Autodesk Inventor part; units mm, degrees
ref_plane "YZ Plane" through (0, 0, 0) normal (1, 0, 0) x (0, 1, 0)
ref_plane "XZ Plane" through (0, 0, 0) normal (0, 1, 0) x (-1, 0, 0)
ref_plane "XY Plane" through (0, 0, 0) normal (0, 0, 1) x (1, 0, 0)
sketch "Sketch1" plane through (0, 0, 0) normal (0, 1, 0) x (-1, 0, 0)
  line L0 (0, 0) -> (304.8, 0)
  line L1 (304.8, 0) -> (304.8, -190.5)
  line L2 (304.8, -190.5) -> (0, -190.5)
  line L3 (0, -190.5) -> (0, 0)
  dimension "d0" = 304.8
  dimension "d1" = 190.5
extrude "Extrusion1" add sketch "Sketch1" along normal blind 1.6
sketch "Sketch2" plane through (0, 1.6, 0) normal (0, 1, 0) x (1, 0, 0)
  line L0 (-304.8, 0) -> (0, 0)
  line L1 (-140.97, 0) -> (-140.97, 10.16)
  line L2 (-140.97, 0) -> (-130.81, 0) construction
  line L3 (-140.97, 10.16) -> (-140.97, 33.02)
  line L4 (-140.97, 33.02) -> (-255.8376, 33.02)
  line L5 (-140.97, 10.16) -> (-95.25, 10.16)
  line L6 (-95.25, 10.16) -> (-16.51, 10.16)
  line L7 (-16.51, 10.16) -> (-16.51, 165.1)
  line L8 (-140.97, 10.16) -> (-140.97, 165.1)
  line L9 (0, 0) -> (0, 190.5)
  line L10 (-16.51, 165.1) -> (-295.91, 165.1)
  line L11 (-295.91, 165.1) -> (-295.91, 33.02)
  line L12 (-295.91, 33.02) -> (-255.8376, 33.02)
  circle A0 centre (-295.91, 33.02) radius 2.54
  circle A1 centre (-295.91, 165.1) radius 2.54
  circle A2 centre (-140.97, 165.1) radius 2.54
  circle A3 centre (-16.51, 165.1) radius 2.54
  circle A4 centre (-16.51, 10.16) radius 2.54
  circle A5 centre (-140.97, 10.16) radius 2.54
  point P0 (-299.72, 0)
  point P1 (-5.08, 0)
  point P2 (0, 5.08)
  point P3 (0, 185.42)
  dimension "d5" = 10.16
  dimension "d6" = 90
  dimension "d8" = 78.74
  dimension "d9" = 45.72
  dimension "d10" = 22.86
  dimension "d11" = 154.94
  dimension "d12" = 154.94
  dimension "d13" = 16.51
  dimension "d14" = 279.4
  dimension "d15" = 5.08
  dimension "d16" = 5.08
  dimension "d17" = 5.08
  dimension "d18" = 5.08
  dimension "d19" = 5.08
  dimension "d20" = 5.08
extrude "Extrusion2" cut sketch "Sketch2" against normal through all contours A5 L3 L1 | L1 L5 A5 | L3 A5 L5 | A2 L10 L8 | L8 L10 A2 | A4 L7 L6 | L6 L7 A4 | A0 L11 L12 | L12 L11 A0 | L10 A2 | A1 L11 L10 | L10 L11 A1 | A3 L7 L10 | L10 L7 A3
sketch "Sketch3" plane through (0, 0, 0) normal (0, 1, 0) x (-1, 0, 0)
  circle A0 centre (16.51, -165.1) radius 2.54
  circle A1 centre (16.51, -165.1) radius 2.3813
  circle A2 centre (16.51, -10.16) radius 2.54
  circle A3 centre (16.51, -10.16) radius 2.3813
  circle A4 centre (140.97, -10.16) radius 2.54
  circle A5 centre (140.97, -10.16) radius 2.3813
  circle A6 centre (295.91, -33.02) radius 2.54
  circle A7 centre (295.91, -33.02) radius 2.3813
  circle A8 centre (295.91, -165.1) radius 2.54
  circle A9 centre (295.91, -165.1) radius 2.3813
  circle A10 centre (140.97, -165.1) radius 2.54
  circle A11 centre (140.97, -165.1) radius 2.3813
  point P0 (0, 0)
extrude "Extrusion3" add sketch "Sketch3" along normal blind 2.54 contours A0 | A1 | A2 | A3 | A4 | A5 | A6 | A7 | A8 | A9 | A10 | A11
sketch "Sketch4" plane through (-140.97, 2.54, -10.16) normal (0, 1, 0) x (1, 0, 0)
  circle A0 centre (0, 0) radius 1.9812
  circle A1 centre (-154.94, 22.86) radius 2.54
  circle A2 centre (-154.94, 22.86) radius 1.9812
  circle A3 centre (0, 154.94) radius 2.54
  circle A4 centre (0, 154.94) radius 1.9812
  circle A5 centre (124.46, 154.94) radius 2.54
  circle A6 centre (124.46, 154.94) radius 1.9812
  circle A7 centre (-154.94, 154.94) radius 2.54
  circle A8 centre (-154.94, 154.94) radius 1.9812
  circle A9 centre (124.46, 0) radius 2.54
  circle A10 centre (124.46, 0) radius 1.9812
  point P0 (140.97, -10.16)
  dimension "d25" = 3.9624
  dimension "d26" = 3.9624
  dimension "d27" = 3.9624
  dimension "d28" = 3.9624
  dimension "d29" = 3.9624
extrude "Extrusion4" add sketch "Sketch4" along normal blind 1.27 contours A0 | A2 | A4 | A6 | A8 | A10
equation "\"d12\" = d11"
equation "\"d16\" = d15"
equation "\"d17\" = d15"
equation "\"d18\" = d15"
equation "\"d19\" = d15"
equation "\"d20\" = d15"
properties part number "MotherboardPlate"
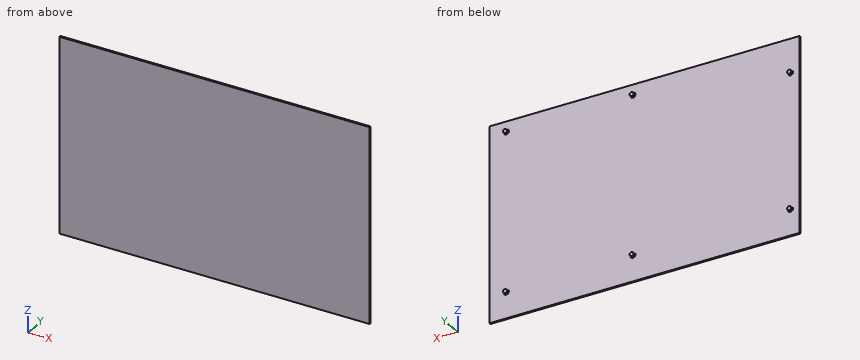
Geometry check sheet. Reference: the model listing, model coordinates, mm. Round coordinates to 2 decimals unless told otherwise and drop trailing zeros. Write each loop counter-clockwise with the first axis right and the second up, starting at its lowest first coordinate (ties: lowest second). Pieces come first, ordered by that corner, then holes.
Item 1: Section check A-A (z = -140). Record the boundary of the cut face in (x, y), plus the area to 3 significant figures.
Determined:
outline: (-304.8, 0) - (0, 0) - (0, 1.6) - (-304.8, 1.6) - close
area: 488 mm2
Item 2: Section check B-B (x = -44). Record the boundary of the cut face in (y, z), plus the area to 3 significant figures.
Determined:
outline: (0, -190.5) - (1.6, -190.5) - (1.6, 0) - (0, 0) - close
area: 305 mm2
Item 3: Material ranges on line 1 along Y through (x, z) = (-207, -84), recorded low to high.
Determined:
line 1: y = 0 to 1.6
Item 4: Go/stop test with a flat-tipped pin: pin 1 Ø1 at (x, z) = (-58.5, -100.5) entering from +Y. Record where the tip stops, or that it passes through.
Determined:
pin 1: stops at y = 1.6
